Here's how the part is built. I have some questions about the finished solid (model axes, mm). A direction names the side the tool comes from. Give positions to 0.01 mm unless a question says otherwise; leave off trailing zeros. Loops run counter-clockwise (first coordinate to the right, second up) from the corner with the lowest first, then second, coordinate; pieces in that order, holes last.
Q1. Suppose I cut it at B-B (y = -5). Count the separate pieces of the cut face and the enclosed holes in it, and give its area (3 significant figures).
Q2. Suppose I cut it at D-D (x = 185). List the corners of the cut face in (y, z) for me.
Q3. I'm going to push flat-ended pins straight in: P1, Ø2, axis at x = 141.5, y = -3, coming from the +Z side; P2, Ø3, axis at x = 169.5, y = -3.5, coming from the -Z side; P3, Ø3, axis at y = -5, z = -25, coming from the +X side; P4, Ø4, axis at x = 177, z = -49, coming from the -Y side. Where does each tip first touch, or does it pass through?
Q4. Suppose I cut it at A-A (z = -108). List the corners of the cut face in (x, y) for me.
Q5. I need wall thicknesses on probe 1 along X at (y, z) = (-3.5, -49); probe 2 along Z at (x, y) = (215, -5); probe 3 along Z at (x, y) = (134, -4.5). Which ranges of each line are inside material? Lowest first, please.
Q6. For faces 4 (the face through (367, -5, 0)), 5 (the face through (300.933, -5.07, -107.325)), 6 (the face through (195, -5, -25)), which set-ups out of +Z, -Z, +X, -X, +Y, -Y let a thin tool reach every point of the face, with its end or its side?
Q7. Thinking about a two-plate mould opening in X: for faces 1 (the face through (300.933, -5.07, -12.675)), 2 (the face through (25, -5, 0)), 3 (the face through (392, -2, -59)), which applies, pulls with the +X half, pulls with the -X half, needs draft (parallel to the pull), parting line crosses it, or undercut?
Q8. Suppose I cut it at C-C (x = 288). List the corners of the cut face in (y, z) for me.
```python
from build123d import *

# Parameters (mm, degrees)
CROQUIS1_W              = 392
CROQUIS1_H              = 120
SALIENTE_EXTRUIR1_DEPTH = 10
CROQUIS2_R              = 2.5
CORTAR_EXTRUIR1_DEPTH   = 411.078041353
CHAFL_N1_SIZE           = 0.5
CROQUIS3_R              = 2.5
CORTAR_EXTRUIR2_DEPTH   = 30
CORTAR_EXTRUIR3_START   = -30
CROQUIS4_R              = 2.5
CORTAR_EXTRUIR3_DEPTH   = 30
CHAFL_N2_SIZE           = 0.5
CORTAR_EXTRUIR4_DEPTH   = 411.078041353


with BuildPart() as part:
    # Croquis1 → Saliente-Extruir1 (new body)
    with BuildSketch(Plane(origin=(0, 0, 0), x_dir=(1, 0, 0), z_dir=(0, 1, 0))):
        with Locations((196, 60)):
            Rectangle(CROQUIS1_W, CROQUIS1_H)
    extrude(amount=-SALIENTE_EXTRUIR1_DEPTH)

    # Croquis2 → Cortar-Extruir1 (cut, through all)
    with BuildSketch(Plane.XZ.offset(10)):
        with Locations(Location((177, -49, 0), (0, 0, 270))):
            Circle(CROQUIS2_R)
        with Locations(Location((177, -71, 0), (0, 0, 270))):
            Circle(CROQUIS2_R)
        with Locations(Location((215, -49, 0), (0, 0, 270))):
            Circle(CROQUIS2_R)
        with Locations(Location((215, -71, 0), (0, 0, 270))):
            Circle(CROQUIS2_R)
    extrude(amount=-CORTAR_EXTRUIR1_DEPTH, mode=Mode.SUBTRACT)

    # Chaflán1
    chafl_n1_edges = [part.edges().sort_by_distance(p)[0] for p in [
        (177, 0, -46.5),
        (177, -10, -46.5),
        (177, 0, -68.5),
        (177, -10, -68.5),
        (215, 0, -46.5),
        (215, -10, -46.5),
        (215, 0, -68.5),
        (215, -10, -68.5),
    ]]
    chamfer(chafl_n1_edges, length=CHAFL_N1_SIZE)

    # Croquis3 → Cortar-Extruir2 (cut)
    with BuildSketch(Plane(origin=(392, 0, 0), x_dir=(0, 0, -1), z_dir=(1, 0, 0))):
        with Locations((25, -5)):
            Circle(CROQUIS3_R)
        with Locations((60, -5)):
            Circle(CROQUIS3_R)
        with Locations((95, -5)):
            Circle(CROQUIS3_R)
    extrude(amount=-CORTAR_EXTRUIR2_DEPTH, mode=Mode.SUBTRACT)

    # Croquis4 → Cortar-Extruir3 (cut)
    with BuildSketch(Plane.ZY.offset(CORTAR_EXTRUIR3_START)):
        with Locations(Location((-25, -5, 0), (0, 0, 180))):
            Circle(CROQUIS4_R)
        with Locations(Location((-60, -5, 0), (0, 0, 180))):
            Circle(CROQUIS4_R)
        with Locations(Location((-95, -5, 0), (0, 0, 180))):
            Circle(CROQUIS4_R)
    extrude(amount=CORTAR_EXTRUIR3_DEPTH, mode=Mode.SUBTRACT)

    # Chaflán2
    chafl_n2_edges = [part.edges().sort_by_distance(p)[0] for p in [
        (392, -5, -22.5),
        (392, -5, -57.5),
        (392, -5, -92.5),
        (0, -5, -22.5),
        (0, -5, -57.5),
        (0, -5, -92.5),
    ]]
    chamfer(chafl_n2_edges, length=CHAFL_N2_SIZE)

    # Croquis5 → Cortar-Extruir4 (cut, through all)
    with BuildSketch(Plane.XZ.offset(10)):
        Polygon((50, 0), (131, -25), (261, -25), (342, 0), align=None)
        Polygon((261, -95), (342, -120), (50, -120), (131, -95), align=None)
    extrude(amount=-CORTAR_EXTRUIR4_DEPTH, mode=Mode.SUBTRACT)


solid = part.part
```
Solutions:
1. separate pieces: 1
1. enclosed holes: 4
1. area: 35,500 mm2
2. outline: (-10, -95) - (0, -95) - (0, -25) - (-10, -25) - close
3. P1: stops at z = -25
3. P2: stops at z = -95
3. P3: stops at x = 362
3. P4: passes through
4. outline: (0, -10) - (88.88, -10) - (88.88, 0) - (0, 0) - close; (303.12, -10) - (392, -10) - (392, 0) - (303.12, 0) - close
5. probe 1: x = 0 to 174.5, 179.5 to 212.5, 217.5 to 392
5. probe 2: z = -95 to -73.5, -68.5 to -51.5, -46.5 to -25
5. probe 3: z = -95 to -25
6. face 4: +Z, +X, -X, +Y, -Y
6. face 5: -Z, +Y, -Y
6. face 6: +Z, +Y, -Y
7. face 1: undercut
7. face 2: needs draft
7. face 3: pulls with the +X half
8. outline: (-10, -103.33) - (0, -103.33) - (0, -16.67) - (-10, -16.67) - close
